Autodesk Inventor part; units mm, degrees
ref_plane "YZ Plane" through (0, 0, 0) normal (1, 0, 0) x (0, 1, 0)
ref_plane "XZ Plane" through (0, 0, 0) normal (0, 1, 0) x (-1, 0, 0)
ref_plane "XY Plane" through (0, 0, 0) normal (0, 0, 1) x (1, 0, 0)
sketch "Skizze1" plane through (0, 0, 0) normal (0, 0, 1) x (1, 0, 0)
  line L0 (-75, 0) -> (75, 0) construction
  circle A0 centre (0, 0) radius 37.5 construction
  line L1 (0, 0) -> (0, 125) construction
  line L2 (0, 125) -> (0, 150) construction
  line L3 (-7.5, 150) -> (7.5, 150) construction
  line L4 (-7.5, 125) -> (7.5, 125) construction
  line L5 (-7.5, 150) -> (7.5, 150)
  line L6 (7.5, 125) -> (7.5, 150)
  line L7 (-7.5, 150) -> (-7.5, 125)
  circle A1 centre (0, 0) radius 45 construction
  line L8 (-7.5, 125) -> (-57.7859, -42.6196)
  line L9 (7.5, 125) -> (57.7859, -42.6196)
  line L10 (-50.6022, -44.7747) -> (0, 123.8992)
  line L11 (0, 123.8992) -> (50.6022, -44.7747)
  line L12 (-57.7859, -42.6196) -> (-50.6022, -44.7747)
  line L13 (57.7859, -42.6196) -> (50.6022, -44.7747)
  point P0 (-45, 0)
  point P1 (45, 0)
  dimension "d0" = 150
  dimension "d1" = 75
  dimension "d2" = 125
  dimension "d3" = 25
  dimension "d4" = 15
  dimension "d5" = 90
  dimension "d6" = 175
  dimension "d7" = 175
  dimension "d8" = 7.5
  dimension "d9" = 7.5
extrude "Extrusion1" add sketch "Skizze1" along normal blind 10
sketch "Skizze2" plane through (0, 0, 10) normal (0, 0, 1) x (1, 0, 0)
  line L0 (-7.5, 150) -> (-7.5, 125)
  line L1 (7.5, 150) -> (-7.5, 150)
  line L2 (7.5, 125) -> (7.5, 150)
  line L3 (-7.5, 125) -> (7.5, 125)
  point P0 (0, 0)
extrude "Extrusion2" add sketch "Skizze2" along normal blind 5
sketch "Skizze3" plane through (0, 0, 10) normal (0, 0, 1) x (1, 0, 0)
  line L0 (-75, 0) -> (75, 0) construction
  line L1 (-50.6022, -44.7747) -> (0, 123.8992)
  line L2 (0, 123.8992) -> (50.6022, -44.7747)
  point P0 (0, 0)
  point P1 (-37.1698, 0)
  point P2 (37.1698, 0)
equation "\"Biegeradius\" = Stärke"
equation "\"BreiteBiegungsfreistellung\" = Stärke"
equation "\"TiefeBiegungsfreistellung\" = 0.5 * Stärke"
equation "\"GrößeEckenfreistellung\" = 4 * Stärke"
equation "\"MinimalRest\" = 2 * Stärke"
equation "\"Übergangsradius\" = Biegeradius"
equation "\"JacobiRadiusGröße\" = Biegeradius"
equation "\"Abstandsgröße\" = Stärke"
properties part number "deichsel"
Verification items for the finished model (mm, model axes). A direction names the side the tool comes from. Coordinates: 2 decimals unless noted, no trailing zeros. Loops run counter-clockwise (first coordinate to the right, second up) from the corner with the lowest first, then second, coordinate; pieces in that order, holes last. Notation, with made-up numbers: M -31,45.5 L 25,45.5 A19 cw 25,61.5 Z; hole C -24,11 d4. An arc over 180 degrees is marked long. One line per item, written item: value.
1. Material ranges on line 1 along Z through (x, y) = (-48, -13.5); line 2 along X through (y, z) = (28.5, 8); line 3 along X through (y, z) = (79, 9.75), recorded low to high. Write a range as from..to.
Answers follow:
line 1: 0..10
line 2: -36.45..-28.62, 28.62..36.45
line 3: -21.3..-13.47, 13.47..21.3
2. Gauge pin test, flat ends, axial feed: P1, Ø1.5, axis at x = -2, z = 11.5, coming from the -Y side; P2, Ø1.5, axis at x = 5.5, y = 106, coming from the +Z side. Record the tip position at first contact, or that the pin passes through.
Answers follow:
P1: y = 125
P2: z = 10
3. Set-up check for faces 1 (the flat face through (0, 125, 12)), 2 (the flat face through (24.947, 40.743, 4.93)), 3 (the flat face through (-7.5, 138, 7)): record each of +Z, -Z, +X, -X, +Y, -Y from which the full face is reachable in a straight line by a thin tool's end or side.
Answers follow:
face 1: +Z, +X, -X, -Y
face 2: +Z, -Z, -Y
face 3: +Z, -Z, -X, +Y
4. Section check A-A on y = -7.5. Record the cut outline in (x, z), plus the area to 3 significant figures.
Answers follow:
outline: M -47.25,0 L -39.42,0 L -39.42,10 L -47.25,10 Z; M 39.42,0 L 47.25,0 L 47.25,10 L 39.42,10 Z
area: 157 mm^2
5. Section check D-D on x = 21. Record the cut outline in (y, z).
Answers follow:
outline: M 53.9,0 L 80,0 L 80,10 L 53.9,10 Z
6. Section check B-B on z = 6.25. Record the cut outline in (x, y), plus the area to 3 significant figures.
Answers follow:
outline: M -57.79,-42.62 L -50.6,-44.77 L 0,123.9 L 50.6,-44.77 L 57.79,-42.62 L 7.5,125 L 7.5,150 L -7.5,150 L -7.5,125 Z
area: 3,020 mm^2
7. Section check C-C on x = 3. Record the cut outline in (y, z), plus the area to 3 significant figures.
Answers follow:
outline: M 113.9,0 L 150,0 L 150,15 L 125,15 L 125,10 L 113.9,10 Z
area: 486 mm^2
